Here's how the part is built. I have some questions about the finished solid (model axes, mm). Coordinates: 2 decimals unless noted, no trailing zeros. Loops run counter-clockwise (first coordinate to the right, second up) from the corner with the lowest first, then second, coordinate; pieces in that order, holes last. Notation, with made-up numbers: M 16,22.25 L 47,22.25 A26 cw 47,55.25 Z; hole C -20,-12.5 d4. An arc over 180 degrees is marked long. Use one line per item in the form item = value. Start each with the question number.
(1) Imagine slicing it at C-C, the plane x = -4. Please give me the cut outline in (y, z).
(2) Will these pins go through, and if not, where does the flat tip stop? P1, Ø1, axis at x = -12.5, z = -1, coming from the -Y side; P2, Ø3, axis at x = -4, z = 9, coming from the +Y side; P3, Ø8, axis at x = -13, z = -16, coming from the -Y side; P4, Ø1, axis at y = 15.5, z = 2, coming from the +X side.
(3) Imagine slicing it at A-A, the plane y = 0. Please give me the cut outline in (x, z), and give its area (3 significant figures).
(4) Please list where these lines run through material, in increasing order: L1, parallel to X at y = 14, z = 10; L2, parallel to Z at x = -4, y = 5.5; L3, parallel to Y at x = -33, z = -6.
(5) Imagine slicing it at D-D, the plane x = -32. Please give me the cut outline in (y, z).
(6) Thinking about a two-plate mould opening in Y: for faces 1 (the flat face through (-10, -6, -6)), 2 (the cylindrical face through (-23.56, -6.84, -0.9)), which applies, +Y half, -Y half, draft (parallel to the pull), parting line (faces both ways), or undercut?
```python
from build123d import *

# Parameters (mm, degrees)
PAD_DEPTH = 10


with BuildPart() as part:
    # Sketch → Revolution (revolve)
    with BuildSketch(Plane.XZ):
        Polygon((-37.5, 6.9), (-10, 6.9), (-10, 20), (0, 20), (0, 0), (-37.5, 0), align=None)
    revolve(axis=Axis((0, 0, 0), (1, 0, 0)))

    # Sketch001 (on Face4 of Revolution) → Pad (new body)
    with BuildSketch(Plane(origin=(0, 0, 0), x_dir=(0, 0, 1), z_dir=(1, 0, 0))):
        with BuildLine():
            ThreePointArc((-21.567608, 4.79146), (-25.041377, 0), (-21.567608, -4.79146))
            ThreePointArc((-18.638676, -11.862528), (-18.477591, -7.653669), (-21.567608, -4.79146))
            ThreePointArc((-18.638676, -11.862528), (-17.706928, -17.706928), (-11.862528, -18.638676))
            ThreePointArc((-4.79146, -21.567608), (-7.653669, -18.477591), (-11.862528, -18.638676))
            ThreePointArc((-4.79146, -21.567608), (0, -25.041377), (4.79146, -21.567608))
            ThreePointArc((11.862528, -18.638676), (7.653669, -18.477591), (4.79146, -21.567608))
            ThreePointArc((11.862528, -18.638676), (17.706928, -17.706928), (18.638676, -11.862528))
            ThreePointArc((21.567608, -4.79146), (18.477591, -7.653669), (18.638676, -11.862528))
            ThreePointArc((21.567608, -4.79146), (25.041377, 0), (21.567608, 4.79146))
            ThreePointArc((18.638676, 11.862528), (18.477591, 7.653669), (21.567608, 4.79146))
            ThreePointArc((18.638676, 11.862528), (17.706928, 17.706928), (11.862528, 18.638676))
            ThreePointArc((4.79146, 21.567608), (7.653669, 18.477591), (11.862528, 18.638676))
            ThreePointArc((4.79146, 21.567608), (0, 25.041377), (-4.79146, 21.567608))
            ThreePointArc((-11.862528, 18.638676), (-7.653669, 18.477591), (-4.79146, 21.567608))
            ThreePointArc((-11.862528, 18.638676), (-17.706928, 17.706928), (-18.638676, 11.862528))
            ThreePointArc((-21.567608, 4.79146), (-18.477591, 7.653669), (-18.638676, 11.862528))
        make_face()
    extrude(amount=-PAD_DEPTH)


solid = part.part
```
Answer:
q1.outline = M -21.57,-4.79 A5.04 cw -18.64,-11.86 A5.04 ccw -11.86,-18.64 A5.04 cw -4.79,-21.57 A5.04 ccw 4.79,-21.57 A5.04 cw 11.86,-18.64 A5.04 ccw 18.64,-11.86 A5.04 cw 21.57,-4.79 A5.04 ccw 21.57,4.79 A5.04 cw 18.64,11.86 A5.04 ccw 11.86,18.64 A5.04 cw 4.79,21.57 A5.04 ccw -4.79,21.57 A5.04 cw -11.86,18.64 A5.04 ccw -18.64,11.86 A5.04 cw -21.57,4.79 A5.04 ccw Z
q2.P1 = -6.88
q2.P2 = 18.54
q2.P3 = -19.18
q2.P4 = 0
q3.outline = M -37.5,-6.9 L -10,-6.9 L -10,-25.04 L 0,-25.04 L 0,25.04 L -10,25.04 L -10,6.9 L -37.5,6.9 Z
q3.area = 880 mm²
q4.L1 = -10 to 0
q4.L2 = -20.18 to 20.18
q4.L3 = -3.41 to 3.41
q5.outline = C 0,0 d13.8
q6.face_1 = draft
q6.face_2 = parting line
